from build123d import *

# Parameters (mm, degrees)
SKETCH1_W           = 469.9
SKETCH1_H           = 292.14
SKETCH1_R           = 6
SKETCH1_W_2         = 52.5
SKETCH1_H_2         = 211.5
BOSS_EXTRUDE1_DEPTH = 10


with BuildPart() as part:
    # Sketch1 → Boss-Extrude1 (new body)
    with BuildSketch(Plane.XY):
        with Locations((213, 105.75)):
            Rectangle(SKETCH1_W, SKETCH1_H)
        with Locations((33.57, -29.046453277)):
            Circle(SKETCH1_R, mode=Mode.SUBTRACT)
        with Locations((69.32, -29.046453277)):
            Circle(SKETCH1_R, mode=Mode.SUBTRACT)
        with Locations((105.07, -29.046453277)):
            Circle(SKETCH1_R, mode=Mode.SUBTRACT)
        with Locations((140.82, -29.046453277)):
            Circle(SKETCH1_R, mode=Mode.SUBTRACT)
        with Locations((176.57, -29.046453277)):
            Circle(SKETCH1_R, mode=Mode.SUBTRACT)
        with Locations((212.32, -29.046453277)):
            Circle(SKETCH1_R, mode=Mode.SUBTRACT)
        with Locations((248.07, -29.046453277)):
            Circle(SKETCH1_R, mode=Mode.SUBTRACT)
        with Locations((283.82, -29.046453277)):
            Circle(SKETCH1_R, mode=Mode.SUBTRACT)
        with Locations((319.57, -29.046453277)):
            Circle(SKETCH1_R, mode=Mode.SUBTRACT)
        with Locations((355.32, -29.046453277)):
            Circle(SKETCH1_R, mode=Mode.SUBTRACT)
        with Locations((391.07, -29.046453277)):
            Circle(SKETCH1_R, mode=Mode.SUBTRACT)
        with Locations((426.82, -29.046453277)):
            Circle(SKETCH1_R, mode=Mode.SUBTRACT)
        with Locations((-2.18, 240.546453277)):
            Circle(SKETCH1_R, mode=Mode.SUBTRACT)
        with Locations((33.57, 240.546453277)):
            Circle(SKETCH1_R, mode=Mode.SUBTRACT)
        with Locations((69.32, 240.546453277)):
            Circle(SKETCH1_R, mode=Mode.SUBTRACT)
        with Locations((105.07, 240.546453277)):
            Circle(SKETCH1_R, mode=Mode.SUBTRACT)
        with Locations((140.82, 240.546453277)):
            Circle(SKETCH1_R, mode=Mode.SUBTRACT)
        with Locations((176.57, 240.546453277)):
            Circle(SKETCH1_R, mode=Mode.SUBTRACT)
        with Locations((212.32, 240.546453277)):
            Circle(SKETCH1_R, mode=Mode.SUBTRACT)
        with Locations((-2.18, -29.046453277)):
            Circle(SKETCH1_R, mode=Mode.SUBTRACT)
        with Locations((248.07, 240.546453277)):
            Circle(SKETCH1_R, mode=Mode.SUBTRACT)
        with Locations((283.82, 240.546453277)):
            Circle(SKETCH1_R, mode=Mode.SUBTRACT)
        with Locations((319.57, 240.546453277)):
            Circle(SKETCH1_R, mode=Mode.SUBTRACT)
        with Locations((355.32, 240.546453277)):
            Circle(SKETCH1_R, mode=Mode.SUBTRACT)
        with Locations((391.07, 240.546453277)):
            Circle(SKETCH1_R, mode=Mode.SUBTRACT)
        with Locations((426.82, 240.546453277)):
            Circle(SKETCH1_R, mode=Mode.SUBTRACT)
        with Locations((34.25, 105.75)):
            Rectangle(SKETCH1_W_2, SKETCH1_H_2, mode=Mode.SUBTRACT)
        with Locations((105.75, 105.75)):
            Rectangle(SKETCH1_W_2, SKETCH1_H_2, mode=Mode.SUBTRACT)
        with Locations((177.25, 105.75)):
            Rectangle(SKETCH1_W_2, SKETCH1_H_2, mode=Mode.SUBTRACT)
        with Locations((248.75, 105.75)):
            Rectangle(SKETCH1_W_2, SKETCH1_H_2, mode=Mode.SUBTRACT)
        with Locations((320.25, 105.75)):
            Rectangle(SKETCH1_W_2, SKETCH1_H_2, mode=Mode.SUBTRACT)
        with Locations((391.75, 105.75)):
            Rectangle(SKETCH1_W_2, SKETCH1_H_2, mode=Mode.SUBTRACT)
    extrude(amount=BOSS_EXTRUDE1_DEPTH)


solid = part.part
Model file for the job. Use its own axes, mm. Give positions to 0.01 mm unless a question says otherwise; leave off trailing zeros. Loops run counter-clockwise (first coordinate to the right, second up) from the corner with the lowest first, then second, coordinate; pieces in that order, holes last. Notation, with made-up numbers: (38, 51.5) - (93, 51.5) arc R22 ccw to (93, 66.5) - close; hole circle Ø7 at (37, 17). An arc over 180 degrees is marked (long way). Use one line per item in the form item = value.
(1) Drill centre lines: L1, parallel to Y at x = 391, z = 5.75; L2, parallel to Y at x = 355.32, z = 5.5; L3, parallel to Y at x = 2, z = 5.5. Where is each one in solid material? Low to high.
Determined:
L1 = -40.32 to -35.05, -23.05 to 0, 211.5 to 234.55, 246.55 to 251.82
L2 = -40.32 to -35.05, -23.05 to 234.55, 246.55 to 251.82
L3 = -40.32 to -33.35, -24.74 to 236.24, 244.85 to 251.82
(2) Cut at C-C (x = 122). Give the cut face in (y, z).
Determined:
outline = (-40.32, 0) - (0, 0) - (0, 10) - (-40.32, 10) - close; (211.5, 0) - (251.82, 0) - (251.82, 10) - (211.5, 10) - close
(3) Cut at A-A (y = 19.5). Give the cut face in (x, z).
Determined:
outline = (-21.95, 0) - (8, 0) - (8, 10) - (-21.95, 10) - close; (60.5, 0) - (79.5, 0) - (79.5, 10) - (60.5, 10) - close; (132, 0) - (151, 0) - (151, 10) - (132, 10) - close; (203.5, 0) - (222.5, 0) - (222.5, 10) - (203.5, 10) - close; (275, 0) - (294, 0) - (294, 10) - (275, 10) - close; (346.5, 0) - (365.5, 0) - (365.5, 10) - (346.5, 10) - close; (418, 0) - (447.95, 0) - (447.95, 10) - (418, 10) - close
(4) Pull direction Y, two halves, no side cores. Call faces 1 (the face through (60.5, 104, 5)), 2 (the face through (447.95, 104, 5)), 3 (the face through (391, 211.5, 5)): pulls with the +Y half, pulls with the -Y half, needs draft (parallel to the pull), parting line crosses it, or undercut.
Determined:
face_1 = undercut
face_2 = needs draft
face_3 = undercut
(5) Cut at D-D (x = -2.18). Give the cut face in (y, z).
Determined:
outline = (-40.32, 0) - (-35.05, 0) - (-35.05, 10) - (-40.32, 10) - close; (-23.05, 0) - (234.55, 0) - (234.55, 10) - (-23.05, 10) - close; (246.55, 0) - (251.82, 0) - (251.82, 10) - (246.55, 10) - close
(6) Cut at B-B (x = 319.57). Give the cut face in (y, z).
Determined:
outline = (-40.32, 0) - (-35.05, 0) - (-35.05, 10) - (-40.32, 10) - close; (-23.05, 0) - (0, 0) - (0, 10) - (-23.05, 10) - close; (211.5, 0) - (234.55, 0) - (234.55, 10) - (211.5, 10) - close; (246.55, 0) - (251.82, 0) - (251.82, 10) - (246.55, 10) - close
(7) Drop flat-ended pins along their axis: P1, Ø19, axis at x = 105.07, y = -29.05, coming from the -Z side; P2, Ø9.5, axis at x = 283.82, y = -29.05, coming from the -Z side. Give the stop position or say it passes through.
Determined:
P1 = 0
P2 = through
